```python
from build123d import *

# Parameters (mm, degrees)
CROQUIS1_R              = 9
SALIENTE_EXTRUIR1_DEPTH = 65
CROQUIS2_W              = 36
CROQUIS2_H              = 18
SALIENTE_EXTRUIR2_DEPTH = 10
MATRIZL1_COUNT          = 3
MATRIZL1_PITCH          = 18.1
MATRIZL1_COUNT_DIR2     = 2
MATRIZL1_PITCH_DIR2     = 18.1


with BuildPart() as part:
    # Croquis1 → Saliente-Extruir1 (new body)
    with BuildSketch(Plane(origin=(0, 0, 0), x_dir=(1, 0, 0), z_dir=(0, 1, 0))):
        with Locations(Location((0, 0, 0), (0, 0, 270))):
            Circle(CROQUIS1_R)
    saliente_extruir1 = extrude(amount=SALIENTE_EXTRUIR1_DEPTH)

    # Croquis2 → Saliente-Extruir2 (add)
    with BuildSketch(Plane(origin=(0, 65, 0), x_dir=(1, 0, 0), z_dir=(0, 1, 0))):
        with Locations((18, 9)):
            Rectangle(CROQUIS2_W, CROQUIS2_H)
    extrude(amount=-SALIENTE_EXTRUIR2_DEPTH)

    # MatrizL1: Saliente-Extruir1 3 × 2
    with Locations(*[(i * MATRIZL1_PITCH, 0, -j * MATRIZL1_PITCH_DIR2) for i in range(MATRIZL1_COUNT) for j in range(MATRIZL1_COUNT_DIR2) if (i, j) != (0, 0)]):
        add(saliente_extruir1)


solid = part.part
```
CAD build for the part. Positions are in the model's coordinates, mm. A direction names the side the tool comes from. Round coordinates to 2 decimals unless told otherwise and drop trailing zeros. Write each loop counter-clockwise with the first axis right and the second up, starting at its lowest first coordinate (ties: lowest second). Pieces come first, ordered by that corner, then holes. Notation, with made-up numbers: (65.5, 68.5) - (95.5, 68.5) arc R5 cw to (95.5, 75.5) - close; hole circle Ø7 at (44.25, 46.25). An arc over 180 degrees is marked (long way). Write item = value, one per line. Start each with the question number.
Q1. Mould opens along X. For faces 3 (the flat face through (36, 0, 0)), 4 (the cylindrical face through (-5.48, 32.04, -25.24)), 5 (the cylindrical face through (42.283, 32.045, -24.733)) say: pulls with the +X half, pulls with the -X half, needs draft (parallel to the pull), parting line crosses it, or undercut.
Q2. Band-saw the part on A-A (y = 5). Give the cut face in (x, z).
Q3. Which spindle directions (+Z, -Z, +X, -X, +Y, -Y) get a long thin tool onto all of the face, cutting with end or side? Do faces 1 (the flat face through (21, 55, -9)), 2 (the flat face through (0, 0, -18)). Say none if no direction does.
Q4. Drop flat-ended pins along their axis: pin 1 (1.5 mm diameter, centred on x = 1, y = 54.5, fed in from -Z); pin 2 (14.5 mm diameter, centred on x = 27, z = -6.5, fed in from -Y); pin 3 (10 mm diameter, centred on x = 11.5, y = 36, fed in from -Z); pin 4 (1.5 mm diameter, centred on y = 41, z = -10.5, fed in from +X). Give the stop position or say it passes through.
Q5. Band-saw the part on C-C (y = 59.5). Give the cut face in (x, z), then the cut area to 3 significant figures.
Q6. Probe L1, parallel to X at y = 7, z = -14; L2, parallel to X at y = 41.5, z = -24; L3, parallel to Z at x = 30.5, y = 50.5. List the from-to ranges inside material, lowest first. Write a range as from..to.
Q7. Band-saw the part on B-B (x = 29). Give the cut face in (y, z), then the cut area to 3 significant figures.
Q8. Band-saw the part on D-D (x = 41.5). Give the cut face in (y, z), then the cut area to 3 significant figures.
Answers below:
q1.face_3 = needs draft
q1.face_4 = undercut
q1.face_5 = undercut
q2.outline = circle Ø18 at (0, -18.1); circle Ø18 at (0, 0); circle Ø18 at (18.1, -18.1); circle Ø18 at (18.1, 0); circle Ø18 at (36.2, -18.1); circle Ø18 at (36.2, 0)
q3.face_1 = -Y
q3.face_2 = +Z, -Z, +X, -X, -Y
q4.pin_1 = -27.1
q4.pin_2 = 0
q4.pin_3 = -26.96
q4.pin_4 = 42.04
q5.outline = (0, -9.1) arc R9 ccw (long way) to (9, -18) - (9.1, -18) arc R9 ccw (long way) to (27.1, -18) - (27.2, -18) arc R9 ccw (long way) to (36, -9.1) - (36, -9) arc R9 ccw (long way) to (27.2, 0) - (27.1, 0) arc R9 ccw to (9.1, 0) - (9, 0) arc R9 ccw (long way) to (0, -9) - close
q5.area = 1,670 mm2
q6.L1 = -8.01..8.01, 10.09..26.11, 28.19..44.21
q6.L2 = -6.8..6.8, 11.3..24.9, 29.4..43
q6.L3 = -25.06..-11.14, -6.96..6.96
q7.outline = (0, -23.5) - (65, -23.5) - (65, 5.4) - (0, 5.4) - (0, -5.4) - (55, -5.4) - (55, -12.7) - (0, -12.7) - close
q7.area = 1,480 mm2
q8.outline = (0, -25.37) - (65, -25.37) - (65, -10.83) - (0, -10.83) - close; (0, -7.27) - (65, -7.27) - (65, 7.27) - (0, 7.27) - close
q8.area = 1,890 mm2
